```python
from build123d import *

# Parameters (mm, degrees)
PAD_DEPTH       = 100
POCKET_DEPTH    = 100
THICKNESS_T     = 3.2
POCKET001_DEPTH = 3.2
SKETCH005_R     = 1.6
SKETCH005_W     = 25
SKETCH005_H     = 32
POCKET002_DEPTH = 5
POCKET003_DEPTH = 5
PAD001_DEPTH    = 3.5
SKETCH008_R     = 1.6
POCKET004_DEPTH = 5
POCKET005_DEPTH = 5
POCKET006_DEPTH = 5
SKETCH011_R     = 1.6
PAD002_DEPTH    = 5
POCKET007_DEPTH = 2.2


with BuildPart() as part:
    # Sketch → Pad (new body, symmetric)
    with BuildSketch(Plane.YZ):
        with BuildLine():
            Line((-95, 0), (95, 0))
            ThreePointArc((95, 0), (88.5403047419, 23.6522969832), (73.3022221559, 42.8606195157))
            Line((35, 75), (73.3022221559, 42.8606195157))
            Line((-35, 75), (35, 75))
            Line((-93.5150551793, 10), (-35, 75))
            ThreePointArc((-93.5150551793, 10), (-94.4647133512, 5.0307659423), (-95, 0))
        make_face()
    extrude(amount=PAD_DEPTH, both=True)

    # Sketch001 → Pocket (cut, symmetric)
    with BuildSketch(Plane.XZ):
        with BuildLine():
            Line((-110, 0), (-110, 75))
            ThreePointArc((110, 75), (0, 106.1145618), (-110, 75))
            Line((110, 75), (110, 0))
            Line((110, 0), (95, 0))
            Line((95, 0), (91.5797985667, 9.3969262079))
            Line((91.5797985667, 9.3969262079), (67.0264978038, 41.980256839))
            Line((35, 75), (67.0264978038, 41.980256839))
            Line((-35, 75), (35, 75))
            Line((-35, 75), (-67.0264978038, 41.980256839))
            Line((-91.5797985667, 9.3969262079), (-67.0264978038, 41.980256839))
            Line((-95, 0), (-91.5797985667, 9.3969262079))
            Line((-110, 0), (-95, 0))
        make_face()
    extrude(amount=POCKET_DEPTH, both=True, mode=Mode.SUBTRACT)

    # Thickness
    thickness_openings = [part.faces().sort_by_distance(p)[0] for p in [
        (0, 0, 75),
    ]]
    offset(amount=THICKNESS_T, openings=thickness_openings, kind=Kind.INTERSECTION)

    # Sketch003 (on Face19 of Thickness) → Pocket001 (cut)
    with BuildSketch(Plane(origin=(0, -59.0046541218, 53.1178552581), x_dir=(1, 0, 0), z_dir=(0, -0.7432085454, 0.6690598314))):
        Polygon((-85, -68.162306919), (-30, 32.3235468044), (30, 32.3235468044), (85, -68.162306919), align=None)
    extrude(amount=-POCKET001_DEPTH, mode=Mode.SUBTRACT)

    # Sketch005 (on Face21 of Pocket001) → Pocket002 (cut)
    with BuildSketch(Plane(origin=(57.8138617322, 0, 56.074800666), x_dir=(-0.6962282131, 0, 0.7178205035), z_dir=(0.7178205035, 0, 0.6962282131))):
        with Locations((3.8648074159, 37.3056555523)):
            Circle(SKETCH005_R)
        with Locations((3.8648074159, -2.6943444477)):
            Circle(SKETCH005_R)
        with Locations((3.8648074159, 17.3056555523)):
            Rectangle(SKETCH005_W, SKETCH005_H)
    extrude(amount=-POCKET002_DEPTH, mode=Mode.SUBTRACT)

    # Sketch006 (on Face26 of Pocket002) → Pocket003 (cut)
    with BuildSketch(Plane(origin=(0, 53.4483679798, 63.6972845582), x_dir=(1, 0, 0), z_dir=(0, 0.6427876097, 0.7660444431))):
        with BuildLine():
            Line((-20, 28.416096279), (20, 28.416096279))
            ThreePointArc((20, -11.583903721), (40, 8.416096279), (20, 28.416096279))
            Line((-20, -11.583903721), (20, -11.583903721))
            ThreePointArc((-20, 28.416096279), (-40, 8.416096279), (-20, -11.583903721))
        make_face()
    extrude(amount=-POCKET003_DEPTH, mode=Mode.SUBTRACT)

    # Sketch007 (on Face13 of Pocket003) → Pad001 (join)
    with BuildSketch(Plane.XY.offset(75)):
        Polygon((-27.4579389755, -39.3056555523), (-27.4579389755, 27.978316246), (27.4579389755, 27.978316246), (27.4579389755, -39.3056555523), (39.4579389755, -39.3056555523), (39.4579389755, 39.978316246), (-39.4579389755, 39.978316246), (-39.4579389755, -39.3056555523), align=None)
    extrude(amount=-PAD001_DEPTH)

    # Sketch008 (on Face41 of Pad001) → Pocket004 (cut)
    with BuildSketch(Plane.XY.offset(75)):
        with Locations((-32.5, 33)):
            Circle(SKETCH008_R)
        with Locations((32.5, 33)):
            Circle(SKETCH008_R)
        with Locations((-32.5, -33)):
            Circle(SKETCH008_R)
        with Locations((32.5, -33)):
            Circle(SKETCH008_R)
    extrude(amount=-POCKET004_DEPTH, mode=Mode.SUBTRACT)

    # Sketch009 (on Face38 of Pocket004) → Pocket005 (cut)
    with BuildSketch(Plane(origin=(65.4833922887, 0, 49.3452754736), x_dir=(0, 1, 0), z_dir=(0.79863551, 0, 0.6018150232))):
        Polygon((-57, -47.0876228441), (-47, -13.5466031816), (-37, -47.0876228441), align=None)
        Polygon((-10, -47.0876228441), (0, -13.5466031816), (10, -47.0876228441), align=None)
        Polygon((37, -47.0876228441), (47, -13.5466031816), (57, -47.0876228441), align=None)
    pocket005 = extrude(amount=-POCKET005_DEPTH, mode=Mode.SUBTRACT)

    # Mirrored: Pocket005 across YZ
    add(pocket005.mirror(Plane.YZ), mode=Mode.SUBTRACT)

    # Sketch010 (on Face55 of Mirrored) → Pocket006 (cut)
    with BuildSketch(Plane(origin=(0, 0, -3.2), x_dir=(1, 0, 0), z_dir=(0, 0, -1))):
        with BuildLine():
            Line((-68.5, -85), (-60.5, -85))
            ThreePointArc((-60.5, -85), (-56.9644660941, -83.5355339059), (-55.5, -80))
            Line((-55.5, -80), (-55.5, 80))
            ThreePointArc((-55.5, 80), (-56.9644660941, 83.5355339059), (-60.5, 85))
            Line((-60.5, 85), (-68.5, 85))
            ThreePointArc((-68.5, 85), (-72.0355339059, 83.5355339059), (-73.5, 80))
            Line((-73.5, 80), (-73.5, -80))
            ThreePointArc((-73.5, -80), (-72.0355339059, -83.5355339059), (-68.5, -85))
        make_face()
        with BuildLine():
            Line((-25.5, -85), (-17.5, -85))
            ThreePointArc((-17.5, -85), (-13.9644660941, -83.5355339059), (-12.5, -80))
            Line((-12.5, -80), (-12.5, 80))
            ThreePointArc((-12.5, 80), (-13.9644660941, 83.5355339059), (-17.5, 85))
            Line((-17.5, 85), (-25.5, 85))
            ThreePointArc((-25.5, 85), (-29.0355339059, 83.5355339059), (-30.5, 80))
            Line((-30.5, 80), (-30.5, -80))
            ThreePointArc((-30.5, -80), (-29.0355339059, -83.5355339059), (-25.5, -85))
        make_face()
        with BuildLine():
            Line((17.5, -85), (25.5, -85))
            ThreePointArc((25.5, -85), (29.0355339059, -83.5355339059), (30.5, -80))
            Line((30.5, -80), (30.5, 80))
            ThreePointArc((30.5, 80), (29.0355339059, 83.5355339059), (25.5, 85))
            Line((25.5, 85), (17.5, 85))
            ThreePointArc((17.5, 85), (13.9644660941, 83.5355339059), (12.5, 80))
            Line((12.5, 80), (12.5, -80))
            ThreePointArc((12.5, -80), (13.9644660941, -83.5355339059), (17.5, -85))
        make_face()
        with BuildLine():
            Line((60.5, -85), (68.5, -85))
            ThreePointArc((68.5, -85), (72.0355339059, -83.5355339059), (73.5, -80))
            Line((73.5, -80), (73.5, 80))
            ThreePointArc((73.5, 80), (72.0355339059, 83.5355339059), (68.5, 85))
            Line((68.5, 85), (60.5, 85))
            ThreePointArc((60.5, 85), (56.9644660941, 83.5355339059), (55.5, 80))
            Line((55.5, 80), (55.5, -80))
            ThreePointArc((55.5, -80), (56.9644660941, -83.5355339059), (60.5, -85))
        make_face()
    extrude(amount=-POCKET006_DEPTH, mode=Mode.SUBTRACT)

    # Sketch011 (on Face64 of Pocket006) → Pad002 (join)
    with BuildSketch(Plane(origin=(-36.6979523749, 13.4389256858, 14.9282978013), x_dir=(0.2975562628, 0.9470000032, -0.1210424075), z_dir=(0.8771991015, -0.3212335505, -0.3568343346))):
        with BuildLine():
            Line((-97.4314518047, 4.7233611651), (-88.7550193505, 15.7106046714))
            Line((-88.7550193505, 15.7106046714), (-96.9132845396, 17.9202899666))
            ThreePointArc((-96.9132845396, 17.9202899666), (-101.098227275, 16.5383837063), (-101.4722817586, 12.1470861926))
            Line((-97.4314518047, 4.7233611651), (-101.4722817586, 12.1470861926))
        make_face()
        with Locations((-97.9590148447, 14.0594030051)):
            Circle(SKETCH011_R, mode=Mode.SUBTRACT)
    pad002 = extrude(amount=-PAD002_DEPTH)

    # Sketch011 (on Face64 of Pocket006) → Pocket007 (cut)
    with BuildSketch(Plane(origin=(-36.6979523749, 13.4389256858, 14.9282978013), x_dir=(0.2975562628, 0.9470000032, -0.1210424075), z_dir=(0.8771991015, -0.3212335505, -0.3568343346))):
        with BuildLine():
            Line((-97.4314518047, 4.7233611651), (-88.7550193505, 15.7106046714))
            Line((-88.7550193505, 15.7106046714), (-96.9132845396, 17.9202899666))
            ThreePointArc((-96.9132845396, 17.9202899666), (-101.098227275, 16.5383837063), (-101.4722817586, 12.1470861926))
            Line((-97.4314518047, 4.7233611651), (-101.4722817586, 12.1470861926))
        make_face()
        with Locations((-97.9590148447, 14.0594030051)):
            Circle(SKETCH011_R, mode=Mode.SUBTRACT)
    pocket007 = extrude(amount=-POCKET007_DEPTH, mode=Mode.SUBTRACT)

    # Mirrored001: Pad002 across YZ
    add(pad002.mirror(Plane.YZ))

    # Mirrored002: Pocket007 across YZ
    add(pocket007.mirror(Plane.YZ), mode=Mode.SUBTRACT)


solid = part.part
```
Input: part model. Units: mm. Frame: model coordinates. A direction names the side the tool comes from. Coordinates: 2 decimals unless noted, no trailing zeros. Write each loop counter-clockwise with the first axis right and the second up, starting at its lowest first coordinate (ties: lowest second). Pieces come first, ordered by that corner, then holes. Notation, with made-up numbers: (84, 85.5) - (112, 85.5) arc R18 ccw to (112, 101.5) - close; hole circle Ø8 at (34.25, 28.5). An arc over 180 degrees is marked (long way). Put each result on its own line as item: value. Start each with the question number.
1) Cut plane B-B (y = 51.5). State how many separate pieces and enclosed holes the cut face has, plus the area to 3 significant figures.
2) Cut plane A-A (x = 84). Return the cut outline in (y, z), plus the area to 3 significant figures.
3) Ray query, L1, parallel to Y at x = -32.5, z = 72.35; L2, parallel to Z at x = 8, y = 70.5; L3, parallel to X at y = 3.5, z = 3.5. Return the intervals inside material, ascending.
4) Reachability of faces 5 (the face through (-57, 83.57, -1.62)), 6 (the face through (-66.26, -79.57, 36.01)), 7 (the face through (57, -83.57, -1.62)) from +Z, -Z, +X, -X, +Y, -Y: full face, straight path, thin tool, end or side. Return the list, or none.
5) Mould query, pull axis Z, two halves, no side actions, for faces 1 (the face through (54.14, -38.89, 57.6)), 2 (the face through (82.33, 4.93, 24.37)), 3 (the face through (29.07, -83.5, -1.62)), 4 (the face through (-82.12, 20.11, 27.27)). Classes: pulls with the +Z half, pulls with the -Z half, needs draft (parallel to the pull), parting line crosses it, or undercut.
6) Cut plane C-C (x = -22.5). Return the cut outline in (y, z), plus the area to 3 significant figures.
7) Contact query for flat-ended pins moving along their axis: pin 1 (2 mm diameter, centred on y = 35.5, z = 62.5, fed in from +X); pin 2 (4 mm diameter, centred on x = 29, z = 9, fed in from +Y); pin 3 (1 mm diameter, centred on y = 19, z = -1, fed in from +X). Output: stop coordinate, or through.
Resolved:
1. separate pieces: 7
1. enclosed holes: 0
1. area: 891 mm2
2. outline: (-98.32, -3.2) - (98.32, -3.2) arc R64.3 ccw to (91.56, 24.77) - (52.13, 24.77) - (53.4, 19.46) - (90.47, 19.46) arc R61.1 cw to (95, 0) - (-95, 0) arc R61.1 cw to (-93.52, 10) - (-85, 19.46) - (-53.4, 19.46) - (-52.13, 24.77) - (-84.52, 24.77) - (-96.44, 11.54) arc R64.3 ccw to start; (-41.87, 24.77) - (-40.6, 19.46) - (-6.4, 19.46) - (-5.13, 24.77) - close; (5.13, 24.77) - (6.4, 19.46) - (40.6, 19.46) - (41.87, 24.77) - close
2. area: 1,540 mm2
3. L1: y = -39.31 to -34.6, -31.4 to 31.4, 34.6 to 43.14
3. L2: z = -3.2 to 0
3. L3: x = -97.13 to -93.73, 93.73 to 97.13
4. face 5: -Z
4. face 6: -X, -Y
4. face 7: +Z, -Z
5. face 1: undercut
5. face 2: undercut
5. face 3: needs draft
5. face 4: pulls with the +Z half
6. outline: (-98.32, -3.2) - (-85, -3.2) - (-85, 0) - (-95, 0) arc R61.1 cw to (-93.52, 10) - (-97.64, 5.41) arc R64.3 ccw to start; (27.98, 71.5) - (39.17, 71.5) - (42.64, 68.59) - (44.69, 71.04) - (39.98, 75) - (27.98, 75) - close; (73.04, 43.08) - (73.3, 42.86) arc R61.1 cw to (95, 0) - (85, 0) - (85, -3.2) - (98.32, -3.2) arc R64.3 ccw to (75.36, 45.31) - (75.1, 45.53) - close
6. area: 331 mm2
7. pin 1: stops at x = 52.55
7. pin 2: stops at y = 97.39
7. pin 3: stops at x = 98.95
